from build123d import *

# Parameters (mm, degrees)
SKETCH1_R           = 1.5
SKETCH1_W           = 4.635083662
SKETCH1_H           = 3
BOSS_EXTRUDE1_DEPTH = 3.5
FILLET1_R           = 2


with BuildPart() as part:
    # Sketch1 → Boss-Extrude1 (new body)
    with BuildSketch(Plane.XY):
        with BuildLine():
            Line((-75.039443802, 3.999805519), (-3.725751189, 4.703060501))
            ThreePointArc((-3.725751189, 4.703060501), (-0.06893841, 5.999603945), (3.616700782, 4.787428898))
            Line((3.616700782, 4.787428898), (35.100171426, 3.998745514))
            ThreePointArc((35.100171426, 3.998745514), (39, 0), (35.100171426, -3.998745514))
            Line((35.100171426, -3.998745514), (3.616700782, -4.787428898))
            ThreePointArc((3.616700782, -4.787428898), (-0.06893841, -5.999603945), (-3.725751189, -4.703060501))
            Line((-3.725751189, -4.703060501), (-75.039443802, -3.999805519))
            ThreePointArc((-75.039443802, -3.999805519), (-79, 0), (-75.039443802, 3.999805519))
        make_face()
        with Locations((-75, 0)):
            Circle(SKETCH1_R, mode=Mode.SUBTRACT)
        Circle(SKETCH1_R, mode=Mode.SUBTRACT)
        with Locations((35, 0)):
            Circle(SKETCH1_R, mode=Mode.SUBTRACT)
        with Locations((-22.682458169, 0)):
            Rectangle(SKETCH1_W, SKETCH1_H, mode=Mode.SUBTRACT)
        with Locations((-47.682458169, 0)):
            Rectangle(SKETCH1_W, SKETCH1_H, mode=Mode.SUBTRACT)
    extrude(amount=BOSS_EXTRUDE1_DEPTH)

    # Fillet1
    fillet1_edges = [part.edges().sort_by_distance(p)[0] for p in [
        (-3.725751189, 4.703060501, 1.75),
        (3.616700782, 4.787428898, 1.75),
        (3.616700782, -4.787428898, 1.75),
        (-3.725751189, -4.703060501, 1.75),
    ]]
    fillet(fillet1_edges, radius=FILLET1_R)


solid = part.part
Verification items for the finished model (mm, model axes). A direction names the side the tool comes from. Give positions to 0.01 mm unless a question says otherwise; leave off trailing zeros. Write each loop counter-clockwise with the first axis right and the second up, starting at its lowest first coordinate (ties: lowest second). Pieces come first, ordered by that corner, then holes.
(1) Cross-section at C-C (x = -42.5). Enter the section's corners in (y, z), plus the area to 3 significant figures.
(2) Material ranges on line 1 (Y direction, x = 0, z = 2.1); line 2 (X direction, y = 1.25, z = 2.9); line 3 (Y direction, x = -75, z = 1.2), recorded low to high.
(3) Access from +Z, -Z, +X, -X, +Y, -Y to the whole of each face (thin tool, end or side, straight path). Record for faces 5 (the face through (-25, 0, 2)), 6 (the face through (-19, 0, 3.5)).
(4) Cross-section at D-D (x = 12.5). Enter the section's corners in (y, z), plus the area to 3 significant figures.
(5) Gauge pin test, flat ends, axial feed: pin 1 (3.5 mm diameter, centred on x = 0, y = 0, fed in from -Z); pin 2 (1.8 mm diameter, centred on x = -23, z = 1.5, fed in from -Y); pin 3 (2 mm diameter, centred on x = 15.5, z = 3, fed in from +Y); pin 4 (2 mm diameter, centred on x = -12.5, z = 2, fed in from +Y). Record the tip position at first contact, or that the pin passes through.
(6) Cross-section at A-A (z = 2.3). Enter the section's corners in (x, y).
(7) Cross-section at B-B (y = 0). Enter the section's corners in (x, z), plus the area to 3 significant figures.
(8) Mould release check, pull along Y, two halves, no side actions. Record for faces 1 (the face through (-19, 0, 0)), 2 (the face through (-23, -1.5, 2)), 3 (the face through (-20.365, 0, 2)), 4 (the face through (39, 0, 2)): +Y half, -Y half, draft (parallel to the pull), parting line (faces both ways), or undercut.
Worked out:
1. outline: (-4.32, 0) - (4.32, 0) - (4.32, 3.5) - (-4.32, 3.5) - close
1. area: 30.2 mm2
2. line 1: y = -6 to -1.5, 1.5 to 6
2. line 2: x = -78.8 to -75.83, -74.17 to -50, -45.36 to -25, -20.36 to -0.83, 0.83 to 34.17, 35.83 to 38.8
2. line 3: y = -4 to -1.5, 1.5 to 4
3. face 5: +Z, -Z
3. face 6: +Z, +X, -X, +Y, -Y
4. outline: (-4.56, 0) - (4.56, 0) - (4.56, 3.5) - (-4.56, 3.5) - close
4. area: 32.0 mm2
5. pin 1: stops at z = 0
5. pin 2: stops at y = -4.52
5. pin 3: stops at y = 4.51
5. pin 4: stops at y = 4.63
6. outline: (-75.04, -4) - (-4.36, -4.7) arc R2 cw to (-3.28, -5.02) arc R6 ccw to (3.19, -5.08) arc R2 cw to (4.21, -4.77) - (35.1, -4) arc R4 ccw to (35.1, 4) - (4.21, 4.77) arc R2 cw to (3.19, 5.08) arc R6 ccw to (-3.28, 5.02) arc R2 cw to (-4.36, 4.7) - (-75.04, 4) arc R4 ccw to start; hole circle Ø3 at (-75, 0); hole (-50, -1.5) - (-45.36, -1.5) - (-45.36, 1.5) - (-50, 1.5) - close; hole (-25, -1.5) - (-20.36, -1.5) - (-20.36, 1.5) - (-25, 1.5) - close; hole circle Ø3 at (0, 0); hole circle Ø3 at (35, 0)
7. outline: (-79, 0) - (-76.5, 0) - (-76.5, 3.5) - (-79, 3.5) - close; (-73.5, 0) - (-50, 0) - (-50, 3.5) - (-73.5, 3.5) - close; (-45.36, 0) - (-25, 0) - (-25, 3.5) - (-45.36, 3.5) - close; (-20.36, 0) - (-1.5, 0) - (-1.5, 3.5) - (-20.36, 3.5) - close; (1.5, 0) - (33.5, 0) - (33.5, 3.5) - (1.5, 3.5) - close; (36.5, 0) - (39, 0) - (39, 3.5) - (36.5, 3.5) - close
7. area: 349 mm2
8. face 1: draft
8. face 2: undercut
8. face 3: undercut
8. face 4: parting line
